from build123d import *

# Parameters (mm, degrees)
PAD004_DEPTH    = 2
SKETCH016_R     = 1.25
POCKET003_DEPTH = 2.001
PAD002_DEPTH    = 2
SKETCH015_R     = 1.25
POCKET002_DEPTH = 2.001
PAD001_DEPTH    = 2
SKETCH017_R     = 1.25
POCKET_DEPTH    = 2.001
SKETCH007_R     = 3
SKETCH008_R     = 1.5
SKETCH005_R     = 3
SKETCH006_R     = 1.5
SKETCH003_R     = 3
SKETCH004_R     = 1.5
SKETCH001_R     = 3
SKETCH002_R     = 1.5
PAD_DEPTH       = 2
PAD003_DEPTH    = 2
SKETCH014_R     = 1.25
POCKET001_DEPTH = 2.001


with BuildPart() as pocket003:
    # Sketch010 → Pad004 (new body)
    with BuildSketch(Plane.XZ.offset(-41.5)):
        Polygon((-38.5, 0), (38.5, 0), (38.5, 8), (28.5, 8), (20, 4), (-20, 4), (-28.5, 8), (-38.5, 8), align=None)
    extrude(amount=PAD004_DEPTH)

    # Sketch016 → Pocket003 (cut, through all)
    with BuildSketch(Plane.XZ.offset(-39.5)):
        with Locations((-35, 4)):
            Circle(SKETCH016_R)
        with Locations((35, 4)):
            Circle(SKETCH016_R)
    extrude(amount=-POCKET003_DEPTH, mode=Mode.SUBTRACT)


with BuildPart() as pocket002:
    # Sketch012 → Pad002 (new body)
    with BuildSketch(Plane.YZ.offset(-41.5)):
        Polygon((-38.5, 0), (38.5, 0), (38.5, 8), (28.5, 8), (20, 4), (-20, 4), (-28.5, 8), (-38.5, 8), align=None)
    extrude(amount=PAD002_DEPTH)

    # Sketch015 → Pocket002 (cut, through all)
    with BuildSketch(Plane.YZ.offset(-39.5)):
        with Locations((-35, 4)):
            Circle(SKETCH015_R)
        with Locations((35, 4)):
            Circle(SKETCH015_R)
    extrude(amount=-POCKET002_DEPTH, mode=Mode.SUBTRACT)


with BuildPart() as pocket:
    # Sketch009 → Pad001 (new body)
    with BuildSketch(Plane.XZ.offset(39.5)):
        Polygon((-38.5, 0), (38.5, 0), (38.5, 8), (28.5, 8), (20, 4), (-20, 4), (-28.5, 7.999908), (-38.5, 7.999908), (-38.5, 8), align=None)
    extrude(amount=PAD001_DEPTH)

    # Sketch017 → Pocket (cut, through all)
    with BuildSketch(Plane.XZ.offset(41.5)):
        with Locations((-35, 4)):
            Circle(SKETCH017_R)
        with Locations((35, 4)):
            Circle(SKETCH017_R)
    extrude(amount=-POCKET_DEPTH, mode=Mode.SUBTRACT)


with BuildPart() as loft003:
    # Sketch007 → Loft003 section 0
    with BuildSketch(Plane.XY):
        with Locations((35, 35)):
            Circle(SKETCH007_R)
    # Sketch008 → Loft003 section 1
    with BuildSketch(Plane.XY.offset(2)):
        with Locations((35, 35)):
            Circle(SKETCH008_R)
    loft(ruled=True)


with BuildPart() as loft002:
    # Sketch005 → Loft002 section 0
    with BuildSketch(Plane.XY):
        with Locations((-35, 35)):
            Circle(SKETCH005_R)
    # Sketch006 → Loft002 section 1
    with BuildSketch(Plane.XY.offset(2)):
        with Locations((-35, 35)):
            Circle(SKETCH006_R)
    loft(ruled=True)


with BuildPart() as loft001:
    # Sketch003 → Loft001 section 0
    with BuildSketch(Plane.XY):
        with Locations((35, -35)):
            Circle(SKETCH003_R)
    # Sketch004 → Loft001 section 1
    with BuildSketch(Plane.XY.offset(2)):
        with Locations((35, -35)):
            Circle(SKETCH004_R)
    loft(ruled=True)


with BuildPart() as loft_body:
    # Sketch001 → Loft section 0
    with BuildSketch(Plane.XY):
        with Locations((-35, -35)):
            Circle(SKETCH001_R)
    # Sketch002 → Loft section 1
    with BuildSketch(Plane.XY.offset(2)):
        with Locations((-35, -35)):
            Circle(SKETCH002_R)
    loft(ruled=True)


with BuildPart() as fusion002:
    # Sketch → Pad (new body)
    with BuildSketch(Plane.XY):
        with BuildLine():
            Line((-41.5, -38.5), (-41.5, 38.5))
            Line((-38.99866, 38.5), (-41.5, 38.5))
            ThreePointArc((-38.99866, 38.5), (-38.645973, 38.646919), (-38.5, 38.999998))
            Line((-38.5, 38.999998), (-38.5, 41.5))
            Line((-38.5, 41.5), (38.5, 41.5))
            Line((38.5, 41.5), (38.5, 38.999998))
            ThreePointArc((38.5, 38.999998), (38.645973, 38.646919), (38.99866, 38.5))
            Line((38.99866, 38.5), (41.5, 38.5))
            Line((41.5, 38.5), (41.5, -38.5))
            Line((39, -38.5), (41.5, -38.5))
            ThreePointArc((39, -38.5), (38.646447, -38.646447), (38.5, -39))
            Line((38.5, -39), (38.5, -41.5))
            Line((-38.5, -41.5), (38.5, -41.5))
            Line((-38.5, -38.998755), (-38.5, -41.5))
            ThreePointArc((-38.5, -38.998755), (-38.633612, -38.658406), (-38.963153, -38.5))
            Line((-38.963153, -38.5), (-41.5, -38.5))
        make_face()
    extrude(amount=PAD_DEPTH)

    # Cut: cut Loft body
    add(loft_body.part, mode=Mode.SUBTRACT)

    # Cut001: cut Loft001
    add(loft001.part, mode=Mode.SUBTRACT)

    # Cut002: cut Loft002
    add(loft002.part, mode=Mode.SUBTRACT)

    # Cut003: cut Loft003
    add(loft003.part, mode=Mode.SUBTRACT)

    # Fusion: union Pocket
    add(pocket.part)

    # Fusion001: union Pocket002
    add(pocket002.part)

    # Fusion002: union Pocket003
    add(pocket003.part)


with BuildPart() as fusion003:
    # Sketch011 → Pad003 (new body)
    with BuildSketch(Plane.YZ.offset(39.5)):
        Polygon((-38.5, 0), (38.5, 0), (38.5, 8), (28.5, 8), (20, 4), (-20, 4), (-28.5, 8), (-38.5, 8), align=None)
    extrude(amount=PAD003_DEPTH)

    # Sketch014 → Pocket001 (cut, through all)
    with BuildSketch(Plane.YZ.offset(41.5)):
        with Locations((-35, 4)):
            Circle(SKETCH014_R)
        with Locations((35, 4)):
            Circle(SKETCH014_R)
    extrude(amount=-POCKET001_DEPTH, mode=Mode.SUBTRACT)

    # Fusion003: union Fusion002
    add(fusion002.part)


solid = fusion003.part
Geometry check sheet. Reference: the model listing, model coordinates, mm. A direction names the side the tool comes from. Give positions to 0.01 mm unless a question says otherwise; leave off trailing zeros. Write each loop counter-clockwise with the first axis right and the second up, starting at its lowest first coordinate (ties: lowest second). Pieces come first, ordered by that corner, then holes. Notation, with made-up numbers: M 2,19 L 12,19 A15 ccw 12,23 Z; hole C 10,-9.75 d9. An arc over 180 degrees is marked long. Answer as CSV lines item,"result". Start each with the question number.
Q1. Section check B-B, the plane z = 7. Give the number of separate pieces and of enclosed holes in the cut face, then the cut area to 3 significant figures.
Q2. Go/stop test with flat-tipped pins: pin 1 (1 mm diameter, centred on x = -24.5, y = 17, fed in from +Z); pin 2 (0.6 mm diameter, centred on x = 41, y = 8, fed in from +Z); pin 3 (0.8 mm diameter, centred on y = 39.5, z = 5.5, fed in from -X). Record where each tip stops, or that it passes through.
Q3. Section check C-C, the plane y = -12.5. Record the cut outline in (x, z).
Q4. Release check for a two-part mould opening along Z. For faces 1 (the face through (40.51, -35.99, 3.24)), 2 (the face through (41, 38.5, 4)), 3 (the face through (-41, 34, 8)) record: pulls with the +Z half, pulls with the -Z half, needs draft (parallel to the pull), parting line crosses it, or undercut.
Q5. Material ranges on L1, parallel to X at y = -23, z = 4; L2, parallel to Z at x = -35, y = -39.9, recorded low to high.
Q6. Section check A-A, the plane x = -35. Record the cut outline in (y, z).
Q7. Tool access check on faces 4 (the face through (38.5, 41, 4)), 5 (the face through (-39.5, -0.5, 3.7)), 6 (the face through (-41, 38.5, 4)), 7 (the face through (-40.51, 24.31, 6.03)). Record the directions out of +Z, -Z, +X, -X, +Y, -Y that give a thin tool (end or side, any length) a straight path to the whole face; none if there is none.
Geometry says:
1,separate pieces,"8"
1,enclosed holes,"0"
1,area,"194 mm^2"
2,pin 1,"z = 2"
2,pin 2,"z = 4"
2,pin 3,"x = -38.5"
3,outline,"M -41.5,0 L 41.5,0 L 41.5,4 L 39.5,4 L 39.5,2 L -39.5,2 L -39.5,4 L -41.5,4 Z"
4,face 1,"undercut"
4,face 2,"needs draft"
4,face 3,"pulls with the +Z half"
5,L1,"-41.5 to -39.5, 39.5 to 41.5"
5,L2,"0 to 2.75, 5.25 to 8"
6,outline,"M -41.5,0 L -38,0 L -36.5,2 L -39.5,2 L -39.5,2.75 L -41.5,2.75 Z; M -41.5,5.25 L -39.5,5.25 L -39.5,8 L -41.5,8 Z; M -33.5,2 L -32,0 L 32,0 L 33.5,2 Z; M 36.5,2 L 38,0 L 41.5,0 L 41.5,2.75 L 39.5,2.75 L 39.5,2 Z; M 39.5,5.25 L 41.5,5.25 L 41.5,8 L 39.5,8 Z"
7,face 4,"+Z, -Z, +X, +Y"
7,face 5,"+Z, +Y, -Y"
7,face 6,"+Z, -Z, -X, +Y"
7,face 7,"+Z, +X, -X"
